```python
from build123d import *

# Parameters (mm, degrees)
SKETCH_1_W          = 76.2
SKETCH_1_H          = 50.8
SKETCH_1_R          = 4.1275
SKETCH_1_R_2        = 4.445
EXTRUDE_1_DEPTH     = 76.2
SKETCH_3_W          = 76.2
SKETCH_3_H          = 76.2
SKETCH_3_R          = 4.7625
EXTRUDE_2_DEPTH     = 50.8
SKETCH_1_4_R        = 4.1275
SKETCH_1_4_R_2      = 4.445
CUT_EXTRUDE_2_DEPTH = 76.2
SKETCH_10_R         = 4.7625
CUT_EXTRUDE_3_DEPTH = 50.8


with BuildPart() as part:
    # Sketch 1 → Extrude 1 (new body)
    with BuildSketch(Plane(origin=(0, 0, 0), x_dir=(0, 0, -1), z_dir=(1, 0, 0))):
        with Locations((38.1, 25.4)):
            Rectangle(SKETCH_1_W, SKETCH_1_H)
        with Locations((38.1, 25.4)):
            Circle(SKETCH_1_R, mode=Mode.SUBTRACT)
        with Locations((25.4, 25.4)):
            Circle(SKETCH_1_R_2, mode=Mode.SUBTRACT)
        with Locations((50.8, 25.4)):
            Circle(SKETCH_1_R_2, mode=Mode.SUBTRACT)
        with Locations((38.1, 38.1)):
            Circle(SKETCH_1_R_2, mode=Mode.SUBTRACT)
        with Locations((38.1, 12.7)):
            Circle(SKETCH_1_R_2, mode=Mode.SUBTRACT)
    extrude(amount=EXTRUDE_1_DEPTH)

    # Sketch 3 → Extrude 2 (add)
    with BuildSketch(Plane(origin=(0, 0, 0), x_dir=(1, 0, 0), z_dir=(0, 1, 0))):
        with Locations((38.1, 38.1)):
            Rectangle(SKETCH_3_W, SKETCH_3_H)
        with Locations((11.0998, 62.5602)):
            Circle(SKETCH_3_R, mode=Mode.SUBTRACT)
        with Locations((65.1002, 13.6398)):
            Circle(SKETCH_3_R, mode=Mode.SUBTRACT)
        with BuildLine():
            Line((17.4498, 45.3898), (17.4498, 13.6398))
            ThreePointArc((17.4498, 13.6398), (11.0998, 7.2898), (4.7498, 13.6398))
            Line((4.7498, 13.6398), (4.7498, 45.3898))
            ThreePointArc((4.7498, 45.3898), (11.0998, 51.7398), (17.4498, 45.3898))
        make_face(mode=Mode.SUBTRACT)
        with BuildLine():
            Line((58.7502, 30.8102), (58.7502, 62.5602))
            ThreePointArc((58.7502, 62.5602), (65.1002, 68.9102), (71.4502, 62.5602))
            Line((71.4502, 62.5602), (71.4502, 30.8102))
            ThreePointArc((71.4502, 30.8102), (65.1002, 24.4602), (58.7502, 30.8102))
        make_face(mode=Mode.SUBTRACT)
    extrude(amount=EXTRUDE_2_DEPTH)

    # Sketch 1_4 → Cut-Extrude 2 (cut)
    with BuildSketch(Plane(origin=(0, 0, 0), x_dir=(0, 0, -1), z_dir=(1, 0, 0))):
        with Locations((38.1, 25.4)):
            Circle(SKETCH_1_4_R)
        with Locations((25.4, 25.4)):
            Circle(SKETCH_1_4_R_2)
        with Locations((50.8, 25.4)):
            Circle(SKETCH_1_4_R_2)
        with Locations((38.1, 38.1)):
            Circle(SKETCH_1_4_R_2)
        with Locations((38.1, 12.7)):
            Circle(SKETCH_1_4_R_2)
    extrude(amount=CUT_EXTRUDE_2_DEPTH, mode=Mode.SUBTRACT)

    # Sketch 10 → Cut-Extrude 3 (cut)
    with BuildSketch(Plane(origin=(0, 0, 0), x_dir=(1, 0, 0), z_dir=(0, 1, 0))):
        with Locations((11.0998, 62.5602)):
            Circle(SKETCH_10_R)
        with Locations((65.1002, 13.6398)):
            Circle(SKETCH_10_R)
        with BuildLine():
            Line((4.7498, 13.6398), (4.7498, 45.3898))
            ThreePointArc((4.7498, 45.3898), (11.0998, 51.7398), (17.4498, 45.3898))
            Line((17.4498, 45.3898), (17.4498, 13.6398))
            ThreePointArc((17.4498, 13.6398), (11.0998, 7.2898), (4.7498, 13.6398))
        make_face()
        with BuildLine():
            Line((71.4502, 62.5602), (71.4502, 30.8102))
            ThreePointArc((71.4502, 30.8102), (65.1002, 24.4602), (58.7502, 30.8102))
            Line((58.7502, 30.8102), (58.7502, 62.5602))
            ThreePointArc((58.7502, 62.5602), (65.1002, 68.9102), (71.4502, 62.5602))
        make_face()
    extrude(amount=CUT_EXTRUDE_3_DEPTH, mode=Mode.SUBTRACT)


solid = part.part
```
The listing builds one solid part. Answer for the finished solid, in the listing's coordinates (mm). A direction names the side the tool comes from. Coordinates: 2 decimals unless noted, no trailing zeros. Write each loop counter-clockwise with the first axis right and the second up, starting at its lowest first coordinate (ties: lowest second). Pieces come first, ordered by that corner, then holes. Notation, with made-up numbers: M 4.5,9 L 42.5,9 A36 cw 42.5,44 Z; hole C -12,57.5 d10. An arc over 180 degrees is marked long. Use a Markdown table: item, result. Add a question column.
1. Section C-C (z = -56.5) is taken. Give the vertices of the cut face in (x, y).
2. Which of the six approach directions +Z, -Z, +X, -X, +Y, -Y give full straight-line access (tool end or side, diameter ignored) to faces 5 (the cylindrical face through (10.96, 30.69, -51.74)), 6 (the cylindrical face through (46.41, 25.6, -20.96))?
3. Section B-B (x = 25.5) is taken. Give the vertices of the cut face in (y, z) (1 decimal), plus the area to 3 significant figures.
4. For a pull along Y with two mould halves and no side action, classify faces 1 (the flat face through (38, 50.8, -38)), 2 (the flat face through (0, 31, -38)), 3 (the flat face through (38, 0, -38)), 4 (the cylindrical face through (2.34, 14.04, -42.34)) as +Y half, -Y half, draft (parallel to the pull), parting line (faces both ways), or undercut.
5. Section A-A (y = 12.7) is taken. Count the separate pieces of the cut face and the enclosed holes in it, plus the area to 3 significant figures.
6. Straight lines are drawn through the part: line 1 along X through (y, z) = (3, -14); line 2 along X through (y, z) = (37, -65); line 3 along X through (y, z) = (4.5, -56). For each, find the intervals that lie inside material, in ascending order. Write a range as [from, to].
7. Section D-D (z = -48) is taken. Give the vertices of the cut face in (x, y).
8. Given P1, Ø8, axis at y = 12.7, z = -38.1, coming from the +X side, flat-ended and moving along its own axis, determine where the tip first touches the part or whether it passes through.
Data:
| question | item | result |
|---|---|---|
| 1 | outline | M 0,0 L 58.75,0 L 58.75,50.8 L 0,50.8 Z; M 71.45,0 L 76.2,0 L 76.2,50.8 L 71.45,50.8 Z |
| 2 | face 5 | +Y, -Y |
| 2 | face 6 | +X, -X |
| 3 | outline | M 0,-76.2 L 50.8,-76.2 L 50.8,0 L 0,0 Z; hole C 12.7,-38.1 d8.9; hole C 25.4,-50.8 d8.9; hole C 25.4,-25.4 d8.9; hole C 25.4,-38.1 d8.3; hole C 38.1,-38.1 d8.9 |
| 3 | area | 3,570 mm2 |
| 4 | face 1 | +Y half |
| 4 | face 2 | draft |
| 4 | face 3 | -Y half |
| 4 | face 4 | undercut |
| 5 | separate pieces | 2 |
| 5 | enclosed holes | 2 |
| 5 | area | 4,150 mm2 |
| 6 | line 1 | x = [0, 4.75], [17.45, 60.35], [69.85, 76.2] |
| 6 | line 2 | x = [0, 7.01], [15.19, 59.24], [70.96, 76.2] |
| 6 | line 3 | x = [0, 58.75], [71.45, 76.2] |
| 7 | outline | M 0,0 L 5.31,0 L 5.31,21.95 L 0,21.95 Z; M 0,28.85 L 5.31,28.85 L 5.31,50.8 L 0,50.8 Z; M 16.89,0 L 58.75,0 L 58.75,21.95 L 16.89,21.95 Z; M 16.89,28.85 L 58.75,28.85 L 58.75,50.8 L 16.89,50.8 Z; M 71.45,0 L 76.2,0 L 76.2,21.95 L 71.45,21.95 Z; M 71.45,28.85 L 76.2,28.85 L 76.2,50.8 L 71.45,50.8 Z |
| 8 | P1 | passes through |
